Input: dimensioned drawing with shaded views. Units: mm. Origin: part minimum x, y, z. Round coordinates to 2 decimals unless told otherwise and drop trailing zeros. Loops run counter-clockwise (first coordinate to the right, second up) from the corner with the lowest first, then second, coordinate; pieces in that order, holes last.
1) First-contact query: pin 1 (12 mm diameter, centred on x = 40, z = 33.5, fed in from -Y); pin 2 (10 mm diameter, centred on x = 26.74, z = 34.03, fed in from -Y). Flat tips, straight axial feed; report the tip coordinate or a pass-through.
2) Section C-C, the plane y = 22. Return loops of the section in (x, z) (1 decimal).
3) Section A-A, the plane x = 30. Return loops of the section in (y, z) (1 decimal).
4) Section B-B, the plane z = 28.5. Return loops of the section in (x, y) (1 decimal), and give its area (3 significant figures).
5) Draft query along X for the marked faces 1, 2, 3 and 4. Return one class per face: pulls with the +X half, pulls with the -X half, needs draft (parallel to the pull), parting line crosses it, or undercut.
6) Ray query, line 1 along X through (y, z) = (19, 33.5) (1 decimal); line 2 along X through (y, z) = (45, 35.5) (1 decimal); line 3 along Z through (x, y) = (21, 39.5) (1 decimal). Return the intervals inside material, ascending.
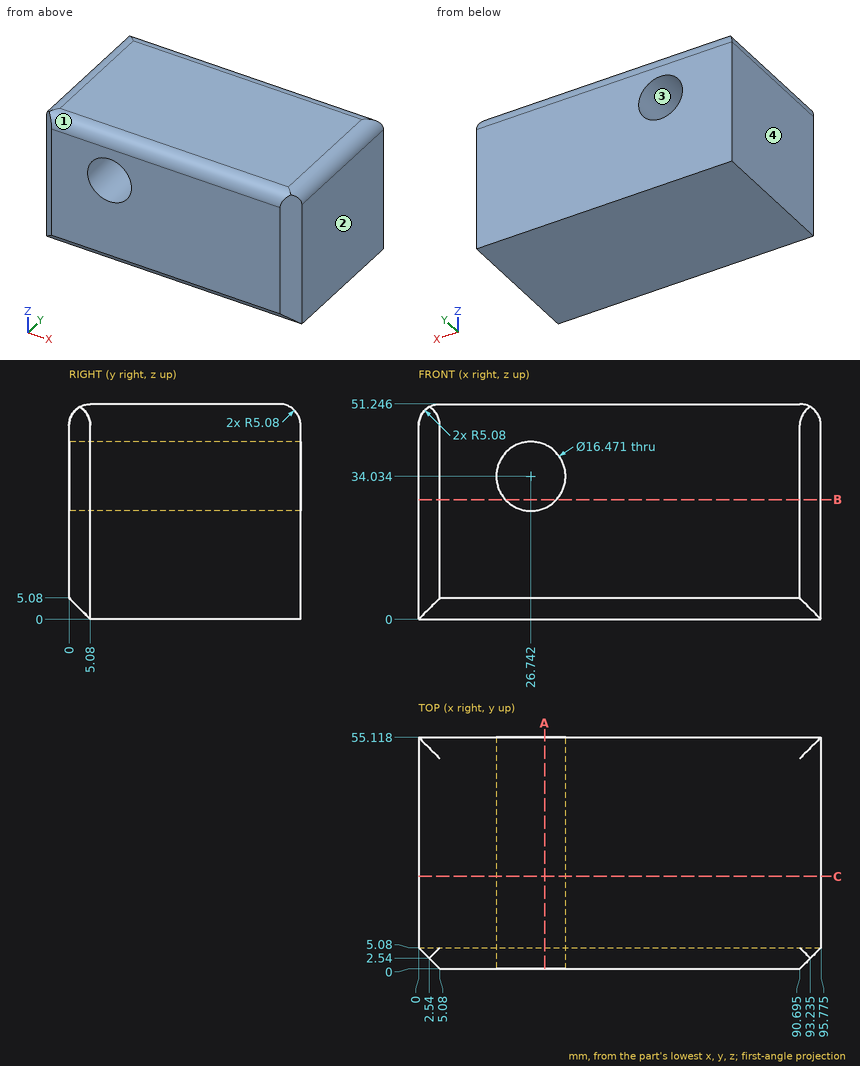
Final values:
1. pin 1: stops at y = 0
1. pin 2: passes through
2. outline: (0, 0) - (95.8, 0) - (95.8, 46.2) arc R5.1 ccw to (90.7, 51.2) - (5.1, 51.2) arc R5.1 ccw to (0, 46.2) - close; hole circle Ø16.5 at (26.7, 34)
3. outline: (0, 5.1) - (5.1, 0) - (55.1, 0) - (55.1, 26.5) - (0, 26.5) - close; (0, 41.6) - (55.1, 41.6) - (55.1, 46.2) arc R5.1 ccw to (50, 51.2) - (5.1, 51.2) arc R5.1 ccw to (0, 46.2) - close
4. outline: (0, 5.1) - (5.1, 0) - (20.6, 0) - (20.6, 55.1) - (0, 55.1) - close; (32.8, 0) - (90.7, 0) - (95.8, 5.1) - (95.8, 55.1) - (32.8, 55.1) - close
4. area: 4,580 mm2
5. face 1: needs draft
5. face 2: pulls with the +X half
5. face 3: undercut
5. face 4: pulls with the -X half
6. line 1: x = 0 to 18.5, 35 to 95.8
6. line 2: x = 0 to 18.6, 34.8 to 95.8
6. line 3: z = 0 to 28.1, 39.9 to 51.2
